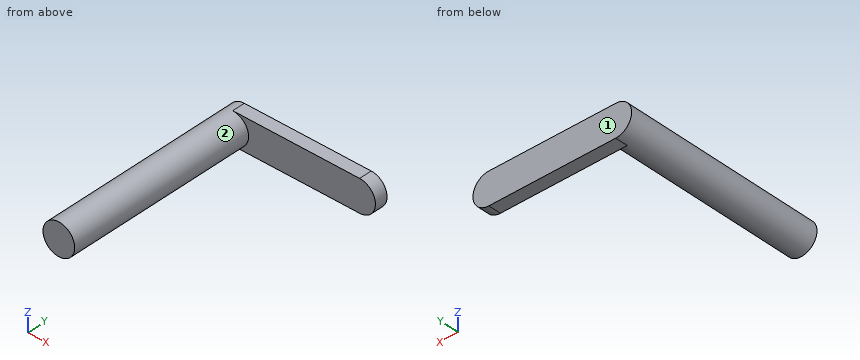
Autodesk Inventor part; units mm, degrees
ref_plane "YZ Plane" through (0, 0, 0) normal (1, 0, 0) x (0, 1, 0)
ref_plane "XZ Plane" through (0, 0, 0) normal (0, 1, 0) x (-1, 0, 0)
ref_plane "XY Plane" through (0, 0, 0) normal (0, 0, 1) x (1, 0, 0)
sketch "Sketch1" plane through (0, 0, 0) normal (0, 1, 0) x (-1, 0, 0)
  circle A0 centre (0, 0) radius 6.35
  dimension "d0" = 12.7
extrude "Extrusion1" add sketch "Sketch1" along normal blind 76.2
sketch "Sketch2" plane through (0, 76.2, 0) normal (0, 1, 0) x (1, 0, 0)
  arc A0 (0, 6.35) -> (0, -6.35) centre (0, 0) ccw
  line L0 (44.45, 0) -> (50.8, 0)
  arc A1 (50.8, -6.35) -> (50.8, 6.35) centre (50.8, 0) ccw
  line L1 (50.8, -6.35) -> (0, -6.35)
  line L2 (0, 6.35) -> (50.8, 6.35)
  dimension "d4" = 6.35
  dimension "d10" = 50.8
  dimension "d11" = 6.35
  dimension "d12" = 50.8
  dimension "d13" = 6.35
extrude "Extrusion2" add sketch "Sketch2" along normal blind 5.08
properties part number "Motor_Arm"
Source: CAD feature listing. Evaluate the final solid. Frame: model axes, mm. Face numbers are marked on the shaded views. A direction names the side the tool comes from. Round coordinates to 2 decimals unless told otherwise and drop trailing zeros. Order: outer loops, then holes, each group sorted by start corner. A loop starts at its lowest first (then second) coordinate and runs counter-clockwise, first axis right, second up. Notation, with made-up numbers: (1.25, 80) -> (54.25, 80) arc R30 ccw to (54.25, 118) -> close; hole circle Ø8 at (57.5, 82). An arc over 180 degrees is marked (long way). One line per item, written item: value. Start each with the question number.
Q1. Material intervals for probe 1 along Y at (x, z) = (13, 4.25); probe 2 along X at (y, z) = (13.5, 0); probe 3 along X at (y, z) = (28, -2.75), sorted ascending.
Q2. Section query C-C (y = 55.5). Return the cut outline in (x, z).
Q3. Access query for the marked faces 1 and 2. Directions: +Z, -Z, +X, -X, +Y, -Y. A direction counts if a zero-diameter tool reaches every point of the face in a straight line with its end or side. Return the directions, or none.
Q4. Section query D-D (z = 4). Return the cut outline in (x, y).
Q5. Section query A-A (x = 45). Return the cut outline in (y, z).
Q6. Pin query (flat end, axial travel): pin 1 (6 mm diameter, centred on y = 59, z = 5, fed in from +X); pin 2 (4 mm diameter, centred on x = 18.5, z = -1.5, fed in from -Y); pin 3 (5 mm diameter, centred on y = 31, z = 1.5, fed in from +X). Return the tip coordinate at first contact, or that it passes through.
Q7. Section query B-B (z = 0). Return the cut outline in (x, y).
Findings below:
1. probe 1: 76.2 to 81.28
1. probe 2: -6.35 to 6.35
1. probe 3: -5.72 to 5.72
2. outline: circle Ø12.7 at (0, 0)
3. face 1: +Z, -Z, +X, -X, +Y
3. face 2: -Y
4. outline: (-4.93, 0) -> (4.93, 0) -> (4.93, 76.2) -> (55.73, 76.2) -> (55.73, 81.28) -> (-4.93, 81.28) -> close
5. outline: (76.2, -6.35) -> (81.28, -6.35) -> (81.28, 6.35) -> (76.2, 6.35) -> close
6. pin 1: x = 6.03
6. pin 2: y = 76.2
6. pin 3: x = 6.35
7. outline: (-6.35, 0) -> (6.35, 0) -> (6.35, 76.2) -> (57.15, 76.2) -> (57.15, 81.28) -> (-6.35, 81.28) -> close
